Autodesk Inventor part; units mm, degrees
ref_plane "YZ Plane" through (0, 0, 0) normal (1, 0, 0) x (0, 1, 0)
ref_plane "XZ Plane" through (0, 0, 0) normal (0, 1, 0) x (-1, 0, 0)
ref_plane "XY Plane" through (0, 0, 0) normal (0, 0, 1) x (1, 0, 0)
sketch "Sketch1" plane through (0, 0, 0) normal (0, 1, 0) x (-1, 0, 0)
  circle A0 centre (0, 0) radius 2
  circle A1 centre (53, 0) radius 2
  arc A2 (53, -5) -> (53, 5) centre (53, 0) ccw
  arc A3 (0, 5) -> (0, -5) centre (0, 0) ccw
  line L0 (31.5, 37.5) -> (31.5, 5)
  line L1 (31.5, -5) -> (31.5, -39)
  line L2 (21.5, 37.5) -> (21.5, 5)
  line L3 (21.5, -5) -> (21.5, -39)
  line L4 (31.5, 39) -> (21.5, 39)
  line L5 (21.5, 39) -> (21.5, 36)
  line L6 (31.5, 36) -> (31.5, 39)
  line L7 (31.5, -39) -> (21.5, -39)
  line L8 (53, 5) -> (31.5, 5)
  line L9 (21.5, 5) -> (0, 5)
  line L10 (53, -5) -> (31.5, -5)
  line L11 (21.5, -5) -> (0, -5)
  dimension "d0" = 4
  dimension "d1" = 4
  dimension "d2" = 10
  dimension "d3" = 10
  dimension "d8" = 3
extrude "Extrusion1" add sketch "Sketch1" along normal blind 3
sketch "Sketch2" plane through (0, 3, 0) normal (0, 1, 0) x (1, 0, 0)
  circle A0 centre (-53, 0) radius 2
  circle A1 centre (0, 0) radius 2
  line L0 (-53, -5) -> (-31.5, -5)
  line L1 (-31.5, -5) -> (-31.5, -39)
  line L2 (-31.5, -39) -> (-21.5, -39)
  line L3 (-21.5, -39) -> (-21.5, -5)
  line L4 (-21.5, -5) -> (0, -5)
  arc A2 (0, -5) -> (0, 5) centre (0, 0) ccw
  line L5 (0, 5) -> (-21.5, 5)
  line L6 (-21.5, 5) -> (-21.5, 39)
  line L7 (-21.5, 39) -> (-31.5, 39)
  line L8 (-31.5, 39) -> (-31.5, 5)
  line L9 (-31.5, 5) -> (-53, 5)
  arc A3 (-53, 5) -> (-53, -5) centre (-53, 0) ccw
  line L10 (-21.5, 5) -> (-21.5, 39)
  line L11 (-31.5, 39) -> (-21.5, 39)
  line L12 (-21.5, 39) -> (-21.5, 36)
  line L13 (-21.5, 36) -> (-31.5, 36)
  line L14 (-31.5, 36) -> (-31.5, 39)
  line L15 (-21.5, -39) -> (-21.5, -5)
  line L16 (-31.5, -39) -> (-21.5, -39)
  line L17 (-21.5, -39) -> (-21.5, -36)
  line L18 (-21.5, -36) -> (-31.5, -36)
  line L19 (-31.5, -36) -> (-31.5, -39)
  dimension "d11" = 3
  dimension "d12" = 3
extrude "Extrusion2" add sketch "Sketch2" along normal blind 15 contours L18 L3 L2 L1 | L8 L7 L6 L13
properties part number "Battery Restraint"
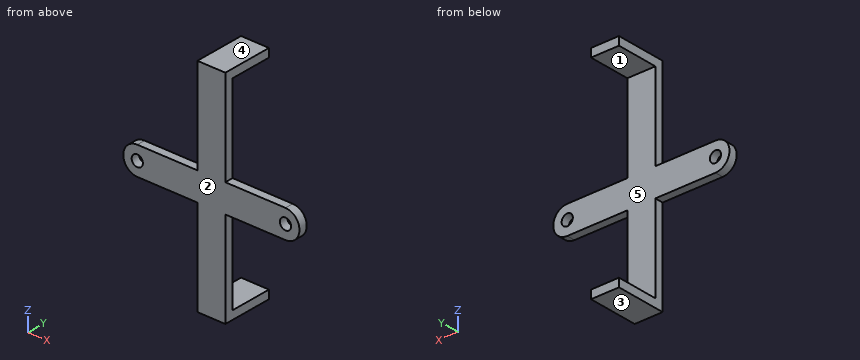
Input: part model. Units: mm. Frame: model coordinates. Face numbers are marked on the shaded views. A direction names the side the tool comes from. Give positions to 0.01 mm unless a question says otherwise; leave off trailing zeros. Order: outer loops, then holes, each group sorted by start corner. A loop starts at its lowest first (then second) coordinate and runs counter-clockwise, first axis right, second up. Notation, with made-up numbers: M -32.75,51 L 5.25,51 A7 cw 5.25,62 Z; hole C 52.25,35.25 d8. An arc over 180 degrees is marked long. Return JSON: item names as keys, results as strings.
Item 1: Ray query, probe 1 along Z at (x, y) = (0, 1.9); probe 2 along Y at (x, z) = (-43.5, -4.5); probe 3 along Z at (x, y) = (-25.5, 8.75). Return the intervals inside material, ascending.
Solutions:
{"probe 1": "-5 to -2, 2 to 5", "probe 2": "0 to 3", "probe 3": "-39 to -36, 36 to 39"}
Item 2: Cut plane A-A (z = 0). Return loops of the section in (x, y).
Solutions:
{"outline": "M -58,0 L -55,0 L -55,3 L -58,3 Z; M -51,0 L -2,0 L -2,3 L -51,3 Z; M 2,0 L 5,0 L 5,3 L 2,3 Z"}
Item 3: First-contact query: P1, Ø5, axis at x = -53, z = 0, coming from the +Y side; P2, Ø9, axis at y = 5, z = 20.5, coming from the +X side; P3, Ø2.5, axis at x = -12, y = 1.5, coming from the +Z side. Flat tips, straight axial feed; report the tip coordinate or a pass-through.
Solutions:
{"P1": "y = 3", "P2": "x = -21.5", "P3": "z = 5"}
Item 4: Cut plane D-D (y = 1.5). Return loops of the section in (x, z), then the cut area to 3 significant figures.
Solutions:
{"outline": "M -53,-5 L -31.5,-5 L -31.5,-39 L -21.5,-39 L -21.5,-5 L 0,-5 A5 ccw 0,5 L -21.5,5 L -21.5,39 L -31.5,39 L -31.5,5 L -53,5 A5 ccw Z; hole C -53,0 d4; hole C 0,0 d4", "area": "1,260 mm^2"}
Item 5: Access query for the marked faces 4 and 5. Directions: +Z, -Z, +X, -X, +Y, -Y. A direction counts if a zero-diameter tool reaches every point of the face in a straight line with its end or side. Return the directions, or none.
Solutions:
{"face 4": "+Z, +X, -X, +Y, -Y", "face 5": "+X, -X, +Y"}
Item 6: Cut plane B-B (y = 8.75). Return loops of the section in (x, z), then the cut area to 3 significant figures.
Solutions:
{"outline": "M -31.5,-39 L -21.5,-39 L -21.5,-36 L -31.5,-36 Z; M -31.5,36 L -21.5,36 L -21.5,39 L -31.5,39 Z", "area": "60.0 mm^2"}
Item 7: Pull-direction query (Z, two-part tool) for the marked faces 1, 2 and 3; classes: +Z half, -Z half, draft (parallel to the pull), parting line (faces both ways), or undercut.
Solutions:
{"face 1": "undercut", "face 2": "draft", "face 3": "-Z half"}
Item 8: Cut plane C-C (x = -23.5). Return loops of the section in (y, z).
Solutions:
{"outline": "M 0,-39 L 18,-39 L 18,-36 L 3,-36 L 3,36 L 18,36 L 18,39 L 0,39 Z"}
